Design review of the part built by this model. Coordinates are the model's own, in mm. Coordinates: 2 decimals unless noted, no trailing zeros. Loops run counter-clockwise (first coordinate to the right, second up) from the corner with the lowest first, then second, coordinate; pieces in that order, holes last. Notation, with made-up numbers: M 7,58 L 38,58 A5 ccw 38,66 Z; hole C 69.5,84.5 d4. An arc over 180 degrees is marked long. Write item = value, one per line. Start each with the question number.
from build123d import *

# Parameters (mm, degrees)
SKETCH1_R           = 3.25
BOSS_EXTRUDE1_DEPTH = 10
CUT_EXTRUDE1_DEPTH  = 7
SKETCH3_R           = 2.5
CUT_EXTRUDE2_DEPTH  = 10
FILLET1_R           = 3.5


with BuildPart() as part:
    # Sketch1 → Boss-Extrude1 (new body)
    with BuildSketch(Plane.XY):
        with BuildLine():
            Line((-73.747603834, 33.92172524), (73.252396166, 33.92172524))
            ThreePointArc((73.252396166, 33.92172524), (76.080823291, 32.750152364), (77.252396166, 29.92172524))
            Line((77.252396166, 29.92172524), (77.252396166, -17.07827476))
            ThreePointArc((77.252396166, -17.07827476), (76.080823291, -19.906701885), (73.252396166, -21.07827476))
            Line((73.252396166, -21.07827476), (-73.747603834, -21.07827476))
            ThreePointArc((-73.747603834, -21.07827476), (-76.576030959, -19.906701885), (-77.747603834, -17.07827476))
            Line((-77.747603834, -17.07827476), (-77.747603834, 29.92172524))
            ThreePointArc((-77.747603834, 29.92172524), (-76.576030959, 32.750152364), (-73.747603834, 33.92172524))
        make_face()
        with Locations((-27.747603834, 3.92172524)):
            Circle(SKETCH1_R, mode=Mode.SUBTRACT)
        with Locations((29.252396166, 0.92172524)):
            Circle(SKETCH1_R, mode=Mode.SUBTRACT)
    extrude(amount=BOSS_EXTRUDE1_DEPTH)

    # Sketch2 → Cut-Extrude1 (cut)
    with BuildSketch(Plane.XY.offset(10)):
        with BuildLine():
            Line((-77.747603834, 20.92172524), (-68.247603834, 20.92172524))
            ThreePointArc((-68.247603834, 20.92172524), (-65.7727301, 21.946851505), (-64.747603834, 24.42172524))
            Line((-64.747603834, 24.42172524), (-64.747603834, 33.92172524))
            Line((-64.747603834, 33.92172524), (-77.747603834, 33.92172524))
            Line((-77.747603834, 33.92172524), (-77.747603834, 20.92172524))
        make_face()
        with BuildLine():
            Line((-77.747603834, -8.07827476), (-68.247603834, -8.07827476))
            ThreePointArc((-68.247603834, -8.07827476), (-65.7727301, -9.103401026), (-64.747603834, -11.57827476))
            Line((-64.747603834, -11.57827476), (-64.747603834, -21.07827476))
            Line((-64.747603834, -21.07827476), (-77.747603834, -21.07827476))
            Line((-77.747603834, -21.07827476), (-77.747603834, -8.07827476))
        make_face()
        with BuildLine():
            Line((64.252396166, -21.07827476), (77.252396166, -21.07827476))
            Line((77.252396166, -21.07827476), (77.252396166, -8.07827476))
            Line((77.252396166, -8.07827476), (67.752396166, -8.07827476))
            ThreePointArc((67.752396166, -8.07827476), (65.277522432, -9.103401026), (64.252396166, -11.57827476))
            Line((64.252396166, -11.57827476), (64.252396166, -21.07827476))
        make_face()
        with BuildLine():
            Line((77.252396166, 20.92172524), (67.752396166, 20.92172524))
            ThreePointArc((67.752396166, 20.92172524), (65.277522432, 21.946851505), (64.252396166, 24.42172524))
            Line((64.252396166, 24.42172524), (64.252396166, 33.92172524))
            Line((64.252396166, 33.92172524), (77.252396166, 33.92172524))
            Line((77.252396166, 33.92172524), (77.252396166, 20.92172524))
        make_face()
    extrude(amount=-CUT_EXTRUDE1_DEPTH, mode=Mode.SUBTRACT)

    # Sketch3 → Cut-Extrude2 (cut)
    with BuildSketch(Plane.XY.offset(3)):
        with Locations((-69.747603834, 25.92172524)):
            Circle(SKETCH3_R)
        with Locations((69.252396166, 25.92172524)):
            Circle(SKETCH3_R)
        with Locations((69.252396166, -13.07827476)):
            Circle(SKETCH3_R)
        with Locations((-69.747603834, -13.07827476)):
            Circle(SKETCH3_R)
    extrude(amount=-CUT_EXTRUDE2_DEPTH, mode=Mode.SUBTRACT)

    # Fillet1
    fillet1_edges = [part.edges().sort_by_distance(p)[0] for p in [
        (64.252396166, 33.92172524, 6.5),
        (77.252396166, 20.92172524, 6.5),
        (77.252396166, -8.07827476, 6.5),
        (64.252396166, -21.07827476, 6.5),
        (-64.747603834, -21.07827476, 6.5),
        (-77.747603834, -8.07827476, 6.5),
        (-77.747603834, 20.92172524, 6.5),
        (-64.747603834, 33.92172524, 6.5),
    ]]
    fillet(fillet1_edges, radius=FILLET1_R)


solid = part.part
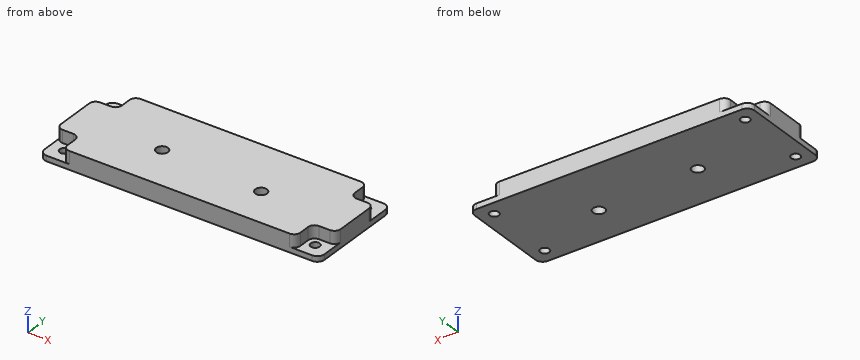
Q1. Add section C-C on y = -1. State the section outline as (x, z) points.
Q2. To check wall thickness, follow line 1 (X direction, y = 3, z = 1); line 2 (X direction, y = 2.5, z = 8.75); line 3 (X direction, y = -15.5, z = 5). State the ranges of each line that lie inside material, in increasing order. Write a range as from..to.
Q3. Add section B-B on z = 7.5. State the section outline as (x, y) points, plus the area to 3 significant figures.
Q4. Clearance check with flat-ended pins moving along their axes: P1, Ø5, axis at x = -71, z = 7.5, coming from the -Y side; P2, Ø5, axis at x = 69.5, z = 8, coming from the -Y side; P3, Ø1, axis at x = 61.5, z = 6, coming from the +Y side; P4, Ø3, axis at x = 69.25, y = -13.08, coming from the +Z side. State where each tip first meets the part, or that it passes through.
Q5. Add section A-A on x = -27.5. State the section outline as (y, z) points.
Values follow:
q1.outline = M -77.75,0 L 26.63,0 L 26.63,10 L -77.75,10 Z; M 31.87,0 L 77.25,0 L 77.25,10 L 31.87,10 Z
q2.line_1 = -77.75..-30.86, -24.63..26.75, 31.75..77.25
q2.line_2 = -77.75..-30.67, -24.83..26.41, 32.09..77.25
q2.line_3 = -64.75..64.25
q3.outline = M -77.75,-4.58 A3.5 ccw -74.25,-8.08 L -68.25,-8.08 A3.5 cw -64.75,-11.58 L -64.75,-17.58 A3.5 ccw -61.25,-21.08 L 60.75,-21.08 A3.5 ccw 64.25,-17.58 L 64.25,-11.58 A3.5 cw 67.75,-8.08 L 73.75,-8.08 A3.5 ccw 77.25,-4.58 L 77.25,17.42 A3.5 ccw 73.75,20.92 L 67.75,20.92 A3.5 cw 64.25,24.42 L 64.25,30.42 A3.5 ccw 60.75,33.92 L -61.25,33.92 A3.5 ccw -64.75,30.42 L -64.75,24.42 A3.5 cw -68.25,20.92 L -74.25,20.92 A3.5 ccw -77.75,17.42 Z; hole C -27.75,3.92 d6.5; hole C 29.25,0.92 d6.5
q3.area = 7,770 mm2
q4.P1 = -8.08
q4.P2 = -8.16
q4.P3 = 33.91
q4.P4 = through
q5.outline = M -21.08,0 L 0.68,0 L 0.68,10 L -21.08,10 Z; M 7.16,0 L 33.92,0 L 33.92,10 L 7.16,10 Z
